Check sheet for the modelled part. Datum: model origin and axes. Units: mm. A direction names the side the tool comes from. Round coordinates to 2 decimals unless told otherwise and drop trailing zeros. Write each loop counter-clockwise with the first axis right and the second up, starting at its lowest first coordinate (ties: lowest second). Pieces come first, ordered by that corner, then holes.
Item 1: Section check A-A, the plane x = 0. Record the cut outline in (y, z).
Item 2: Set-up check for faces 1 (the cylindrical face through (1.43, -0.45, -6.88)), 2 (the cylindrical face through (-2.5, -0.1, 8.8)), 3 (the flat face through (0, 2.25, -4)), 4 (the cylindrical face through (-2.5, -0.1, -8.7)): record each of +Z, -Z, +X, -X, +Y, -Y from which the full face is reachable in a straight line by a thin tool's end or side.
Item 3: Section check C-C, the plane z = -4. Record the cut outline in (x, y), plus the area to 4 significant figures.
Item 4: Material ranges on line 1 along Z through (x, y) = (1.45, 0.7); line 2 along Z through (x, y) = (-1.65, -2.1); line 3 along Z through (x, y) = (-2.2, 1.05), recorded low to high.
Item 5: Section check D-D, the plane z = 0.5. Record the cut outline in (x, y).
Item 6: Depth check by flat-ended pin: pin 1 (0.8 mm diameter, centred on x = 1, z = 3.5, fed in from -Y); pin 2 (0.8 mm diameter, centred on y = 0, z = 4.5, fed in from +X); pin 3 (2 mm diameter, centred on x = 1, z = -1, fed in from -Y). Enter the tip coordinate at first touch or a pass-through.
from build123d import *

# Parameters (mm, degrees)
SKETCH2_W           = 4
SKETCH2_H           = 4
BOSS_EXTRUDE1_DEPTH = 10.6
SKETCH4_W           = 4.5
SKETCH4_H           = 4.5
BOSS_EXTRUDE3_DEPTH = 2.7


with BuildPart() as part:
    # Sketch1 → Revolve1 (revolve)
    with BuildSketch(Plane(origin=(0, 0, 0), x_dir=(0, 0, -1), z_dir=(1, 0, 0)), mode=Mode.PRIVATE) as revolve1_sk:
        Polygon((-9, 0), (9, 0), (9, 2.5), (8.5, 2.5), (8.5, 1.5), (5.3, 1.5), (5.3, 2), (-5.3, 2), (-5.3, 1.5), (-8.5, 1.5), (-8.5, 2.5), (-9, 2.5), align=None)
    revolve(revolve1_sk.sketch.rotate(Axis((0, 0, 9), (0, 0, -1)), 90), axis=Axis((0, 0, 9), (0, 0, -1)))

    # Sketch2 → Boss-Extrude1 (add)
    with BuildSketch(Plane.XY.offset(5.3)):
        Rectangle(SKETCH2_W, SKETCH2_H)
    extrude(amount=-BOSS_EXTRUDE1_DEPTH)

    # Sketch4 → Boss-Extrude3 (add)
    with BuildSketch(Plane.XY.offset(5.3)):
        Rectangle(SKETCH4_W, SKETCH4_H)
    boss_extrude3 = extrude(amount=-BOSS_EXTRUDE3_DEPTH)

    # Mirror1: Boss-Extrude3 across plane
    add(boss_extrude3.mirror(Plane.XY))


solid = part.part
Values found:
1. outline: (-2.5, -9) - (2.5, -9) - (2.5, -8.5) - (1.5, -8.5) - (1.5, -5.3) - (2.25, -5.3) - (2.25, -2.6) - (2, -2.6) - (2, 2.6) - (2.25, 2.6) - (2.25, 5.3) - (1.5, 5.3) - (1.5, 8.5) - (2.5, 8.5) - (2.5, 9) - (-2.5, 9) - (-2.5, 8.5) - (-1.5, 8.5) - (-1.5, 5.3) - (-2.25, 5.3) - (-2.25, 2.6) - (-2, 2.6) - (-2, -2.6) - (-2.25, -2.6) - (-2.25, -5.3) - (-1.5, -5.3) - (-1.5, -8.5) - (-2.5, -8.5) - close
2. face 1: none
2. face 2: +Z
2. face 3: +X, -X, +Y
2. face 4: -Z
3. outline: (-2.25, -2.25) - (2.25, -2.25) - (2.25, 2.25) - (-2.25, 2.25) - close
3. area: 20.25 mm2
4. line 1: z = -9 to -8.5, -5.3 to 5.3, 8.5 to 9
4. line 2: z = -5.3 to -2.6, 2.6 to 5.3
4. line 3: z = -9 to -8.5, -5.3 to -2.6, 2.6 to 5.3, 8.5 to 9
5. outline: (-2, -2) - (2, -2) - (2, 2) - (-2, 2) - close
6. pin 1: stops at y = -2.25
6. pin 2: stops at x = 2.25
6. pin 3: stops at y = -2
